For this review, take the finished solid that the model builds, in its own axes (mm). A direction names the side the tool comes from. Round coordinates to 2 decimals unless told otherwise and drop trailing zeros. Loops run counter-clockwise (first coordinate to the right, second up) from the corner with the lowest first, then second, coordinate; pieces in that order, holes last. Notation, with made-up numbers: (-18.75, 16.25) -> (-4.75, 16.25) arc R29 ccw to (-4.75, 47.25) -> close; hole circle Ø11 at (78.5, 78). An arc over 180 degrees is marked (long way). Use one line per item in the form item = value. Start each with the question number.
from build123d import *

# Parameters (mm, degrees)
BOSS_EXTRUDE1_DEPTH    = 3.175
F_10_CLEARANCE_HOLE1_D = 4.9784
SKETCH5_W              = 12.7
SKETCH5_H              = 44.45
BOSS_EXTRUDE2_DEPTH    = 3.175
F_8_CLEARANCE_HOLE1_D  = 4.3053


with BuildPart() as part:
    # Sketch1 → Boss-Extrude1 (new body)
    with BuildSketch(Plane.XY):
        Polygon((-266.700000508, -12.7), (-266.700000508, 57.15), (-279.400000508, 57.15), (-311.150000508, 57.15), (-330.200000508, 38.1), (-330.200000508, 12.7), (-330.200000508, -12.7), (-279.400000508, -12.7), align=None)
    extrude(amount=BOSS_EXTRUDE1_DEPTH)

    # #10 Clearance Hole1 (through all)
    with Locations(Plane.XY.offset(3.175)):
        with Locations((-273.050000508, 50.8), (-273.050000508, 25.4), (-273.050000508, 0), (-317.500000508, 0), (-292.100000508, 0)):
            Hole(F_10_CLEARANCE_HOLE1_D / 2)

    # Sketch5 → Boss-Extrude2 (add)
    with BuildSketch(Plane.XY.offset(3.175)):
        with Locations((-304.800000508, 34.925)):
            Rectangle(SKETCH5_W, SKETCH5_H)
    extrude(amount=BOSS_EXTRUDE2_DEPTH)

    # #8 Clearance Hole1 (through all)
    with Locations(Plane.XY.offset(6.35)):
        with Locations((-304.800000508, 42.8625), (-304.800000508, 52.3875), (-304.800000508, 33.3375), (-304.800000508, 23.8125)):
            Hole(F_8_CLEARANCE_HOLE1_D / 2)


solid = part.part
Item 1: Take a section at D-D on y = 0. Give the boundary of the cut face in (x, z) (3 decimals).
Item 2: Wall thickness on line 1 (Y direction, x = -304.8, z = 2.5); line 2 (Y direction, x = -292.1, z = 0.85); line 3 (X direction, y = 33.5, z = 5.5): over which ranges is each line inside the solid? List them lowest first.
Item 3: Machinability: for faces 1 (the flat face through (-298.45, 35, 5)), 2 (the flat face through (-311.15, 35, 5)), 3 (the flat face through (-330.2, 13, 2)), which of the approach directions +Z, -Z, +X, -X, +Y, -Y give a long, thin tool a straight path to every point of the face, cutting with its end or side? Answer none if there is none.
Item 4: For P1, Ø3.5, axis at y = 32.5, z = 5.5, coming from the -X side; P2, Ø2.5, axis at y = 43, z = 5, coming from the +X side; P3, Ø8, axis at x = -273.05, y = 25.4, coming from the +Z side (3 decimals), all flat-tipped, find the tip position at first contact; note any pin that passes through.
Item 5: Take a section at B-B on x = -273.05. Give the boundary of the cut face in (y, z) (3 decimals).
Item 6: Take a section at A-A on x = -317.5. Give the boundary of the cut face in (y, z) (3 decimals).
Item 7: Draft analysis for pull direction Y (two halves, no side actions). For faces 4 (the flat face through (-299, -12.7, 2)), 5 (the cylindrical face through (-270.563, 25.509, 1.565)), 6 (the flat face through (-292, 23, 3.175)), state which applies: +Y half, -Y half, draft (parallel to the pull), parting line (faces both ways), or undercut.
Item 8: Take a section at C-C on x = -304.8. Give the boundary of the cut face in (y, z) (3 decimals).
Results:
q1.outline = (-330.2, 0) -> (-319.989, 0) -> (-319.989, 3.175) -> (-330.2, 3.175) -> close; (-315.011, 0) -> (-294.589, 0) -> (-294.589, 3.175) -> (-315.011, 3.175) -> close; (-289.611, 0) -> (-275.539, 0) -> (-275.539, 3.175) -> (-289.611, 3.175) -> close; (-270.561, 0) -> (-266.7, 0) -> (-266.7, 3.175) -> (-270.561, 3.175) -> close
q2.line_1 = -12.7 to 21.66, 25.97 to 31.18, 35.49 to 40.71, 45.02 to 50.23, 54.54 to 57.15
q2.line_2 = -12.7 to -2.49, 2.49 to 57.15
q2.line_3 = -311.15 to -306.95, -302.65 to -298.45
q3.face_1 = +Z, +X, +Y, -Y
q3.face_2 = +Z, -X, +Y, -Y
q3.face_3 = +Z, -Z, -X, +Y, -Y
q4.P1 = -311.15
q4.P2 = -298.45
q4.P3 = 3.175
q5.outline = (-12.7, 0) -> (-2.489, 0) -> (-2.489, 3.175) -> (-12.7, 3.175) -> close; (2.489, 0) -> (22.911, 0) -> (22.911, 3.175) -> (2.489, 3.175) -> close; (27.889, 0) -> (48.311, 0) -> (48.311, 3.175) -> (27.889, 3.175) -> close; (53.289, 0) -> (57.15, 0) -> (57.15, 3.175) -> (53.289, 3.175) -> close
q6.outline = (-12.7, 0) -> (-2.489, 0) -> (-2.489, 3.175) -> (-12.7, 3.175) -> close; (2.489, 0) -> (50.8, 0) -> (50.8, 3.175) -> (2.489, 3.175) -> close
q7.face_4 = -Y half
q7.face_5 = undercut
q7.face_6 = draft
q8.outline = (-12.7, 0) -> (21.66, 0) -> (21.66, 6.35) -> (12.7, 6.35) -> (12.7, 3.175) -> (-12.7, 3.175) -> close; (25.965, 0) -> (31.185, 0) -> (31.185, 6.35) -> (25.965, 6.35) -> close; (35.49, 0) -> (40.71, 0) -> (40.71, 6.35) -> (35.49, 6.35) -> close; (45.015, 0) -> (50.235, 0) -> (50.235, 6.35) -> (45.015, 6.35) -> close; (54.54, 0) -> (57.15, 0) -> (57.15, 6.35) -> (54.54, 6.35) -> close
